Work out the finished part from the listing and answer in its coordinate system (mm). A direction names the side the tool comes from. Give positions to 0.01 mm unless a question says otherwise; leave off trailing zeros. Loops run counter-clockwise (first coordinate to the right, second up) from the corner with the lowest first, then second, coordinate; pieces in that order, holes last. Notation, with made-up numbers: M 47,18 L 52,18 A25 cw 52,49 Z; hole C 9.5,79 d4. An arc over 180 degrees is marked long. Answer in a Markdown table with one row per item. Add a question column.
from build123d import *

# Parameters (mm, degrees)
FILLET2_R     = 0.75
CHAMFER1_SIZE = 0.254


with BuildPart() as part:
    # Sketch1 → Revolve1 (revolve)
    with BuildSketch(Plane(origin=(0, 0, 0), x_dir=(1, 0, 0), z_dir=(0, 1, 0))):
        with BuildLine():
            Line((6.35, 10.16), (-31.636489348, 10.16))
            ThreePointArc((-31.636489348, 10.16), (-33.432540572, 9.416051224), (-34.176489348, 7.62))
            Line((-34.176489348, 7.62), (-34.176489348, 0))
            Line((-34.176489348, 0), (-82.55, 0))
            Line((-82.55, 0), (-82.55, 4.7625))
            Line((-82.55, 4.7625), (-57.15, 4.7625))
            Line((-57.15, 4.7625), (-57.15, 6.5))
            Line((-57.15, 6.5), (-38.1, 6.5))
            Line((-38.1, 6.5), (-38.1, 16.51))
            Line((-38.1, 16.51), (-34.925, 16.51))
            Line((-34.925, 16.51), (-34.925, 15.24))
            ThreePointArc((-34.925, 15.24), (-34.181051224, 13.443948776), (-32.385, 12.7))
            Line((-32.385, 12.7), (6.35, 12.7))
            Line((6.35, 12.7), (6.35, 10.16))
        make_face()
    revolve(axis=Axis((0, 0, 0), (-1, 0, 0)))

    # Fillet2
    fillet2_edges = [part.edges().sort_by_distance(p)[0] for p in [
        (-57.15, 0, 4.7625),
        (-38.1, 0, 6.5),
    ]]
    fillet(fillet2_edges, radius=FILLET2_R)

    # Chamfer1
    chamfer1_edges = [part.edges().sort_by_distance(p)[0] for p in [
        (-57.15, 0, 6.5),
        (-38.1, 0, 16.51),
        (-34.925, 0, 16.51),
        (6.35, 0, 12.7),
        (6.35, 0, 10.16),
        (-82.55, 0, 4.7625),
    ]]
    chamfer(chamfer1_edges, length=CHAMFER1_SIZE)


solid = part.part
(1) The mould has two halves that part along Z. Classify faces 4 (the face through (-82.55, 0, 0)), 5 (the face through (-13.034, -10.074, 1.323)), 6 (the face through (-69.93, 2.9, 3.78)): pulls with the +Z half, pulls with the -Z half, needs draft (parallel to the pull), parting line crosses it, or undercut.
(2) Section A-A, the plane x = -11.5 is taken. Determine the outline of the cut face in (y, z), and give its area (3 significant figures).
(3) Consider line 1 along Y through (x, z) = (-14.5, 0); line 2 along Z through (x, y) = (-26.5, 6). Determine where each line is inside the solid, lowest interval first. Write a range as from..to.
(4) Which of the six approach directions +Z, -Z, +X, -X, +Y, -Y give full straight-line access (tool end or side, diameter ignored) to faces 1 (the face through (-47.747, 3.955, 5.158)), 2 (the face through (-34.925, -15, -5)), 3 (the face through (6.35, 8, 7))?
(5) Each of these flat-tipped pins is pushed along its axis until it touches: P1, Ø5, axis at x = -33, y = -6, coming from the +Z side; P2, Ø3, axis at x = -22.5, y = 10, coming from the +Z side; P3, Ø8, axis at x = -16, z = -13, coming from the -Y side. Where does it stop, or does it pass through?
(6) Section B-B, the plane x = -52 is taken. Determine the outline of the cut face in (y, z).
Numbers:
| question | item | result |
|---|---|---|
| 1 | face 4 | needs draft |
| 1 | face 5 | undercut |
| 1 | face 6 | parting line crosses it |
| 2 | outline | C 0,0 d25.4; hole C 0,0 d20.32 |
| 2 | area | 182 mm² |
| 3 | line 1 | y = -12.7..-10.16, 10.16..12.7 |
| 3 | line 2 | z = -11.19..-8.2, 8.2..11.19 |
| 4 | face 1 | -X |
| 4 | face 2 | +X |
| 4 | face 3 | +Z, -Z, +X, +Y, -Y |
| 5 | P1 | stops at z = 15.8 |
| 5 | P2 | stops at z = 9.44 |
| 5 | P3 | stops at y = -8.96 |
| 6 | outline | C 0,0 d13 |
